Verification items for this drawing (mm, ordinates from the low corner). A direction names the side the tool comes from. Round coordinates to 2 decimals unless told otherwise and drop trailing zeros. Order: outer loops, then holes, each group sorted by start corner. A loop starts at its lowest first (then second) coordinate and runs counter-clockwise, first axis right, second up. Notation, with made-up numbers: (-24.75, 0) -> (25.25, 0) arc R23 cw to (25.25, 17) -> close; hole circle Ø9 at (46.5, 23). An arc over 180 degrees is marked (long way). Answer in a Markdown table with one row per item.
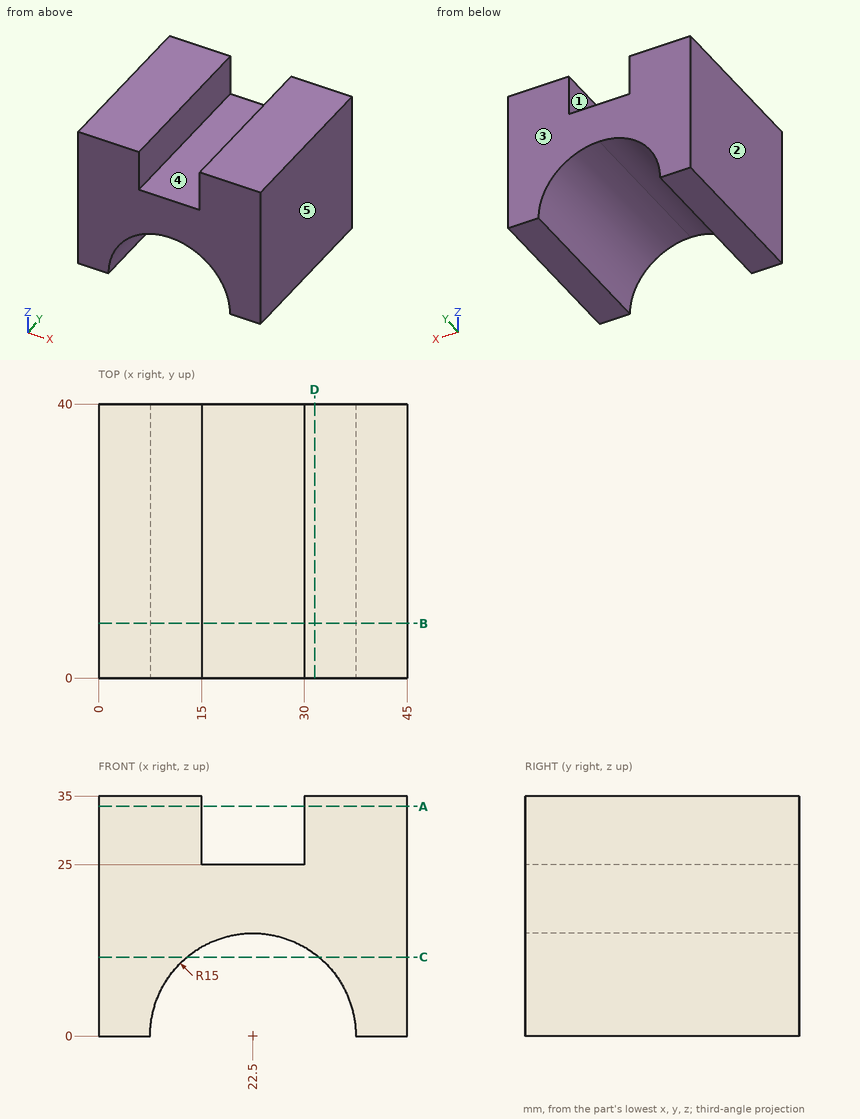
Item 1: Cross-section at D-D (x = 31.5). Record the boundary of the cut face in (y, z), and give its area (3 significant figures).
Result sheet:
| item | result |
|---|---|
| outline | (0, 12) -> (40, 12) -> (40, 35) -> (0, 35) -> close |
| area | 920 mm^2 |
Item 2: Depth check by flat-ended pin: P1, Ø8, axis at x = 35, y = 23, coming from the -Z side; P2, Ø6, axis at x = 14.5, y = 24, coming from the -Z side. Enter the tip coordinate at first touch or a pass-through.
Result sheet:
| item | result |
|---|---|
| P1 | stops at z = 0 |
| P2 | stops at z = 10.2 |
Item 3: Cross-section at A-A (z = 33.5). Record the boundary of the cut face in (x, y), and give its area (3 significant figures).
Result sheet:
| item | result |
|---|---|
| outline | (0, 0) -> (15, 0) -> (15, 40) -> (0, 40) -> close; (30, 0) -> (45, 0) -> (45, 40) -> (30, 40) -> close |
| area | 1,200 mm^2 |
Item 4: Cross-section at B-B (y = 8). Record the boundary of the cut face in (x, z).
Result sheet:
| item | result |
|---|---|
| outline | (0, 0) -> (7.5, 0) arc R15 cw to (22.5, 15) arc R15 cw to (37.5, 0) -> (45, 0) -> (45, 35) -> (30, 35) -> (30, 25) -> (15, 25) -> (15, 35) -> (0, 35) -> close |
Item 5: Scan lines: line 1 (X direction, y = 27.5, z = 31); line 2 (X direction, y = 22, z = 7.5); line 3 (Z direction, x = 23, y = 20). Record each from-to range of solid material in increasing order. Write a range as [from, to].
Result sheet:
| item | result |
|---|---|
| line 1 | x = [0, 15], [30, 45] |
| line 2 | x = [0, 9.51], [35.49, 45] |
| line 3 | z = [14.99, 25] |
Item 6: Mould release check, pull along X, two halves, no side actions. Record for the marked faces 3, 4 and 5: pulls with the +X half, pulls with the -X half, needs draft (parallel to the pull), parting line crosses it, or undercut.
Result sheet:
| item | result |
|---|---|
| face 3 | needs draft |
| face 4 | undercut |
| face 5 | pulls with the +X half |
Item 7: Set-up check for the marked faces 1 and 2: record each of +Z, -Z, +X, -X, +Y, -Y from which the full face is reachable in a straight line by a thin tool's end or side.
Result sheet:
| item | result |
|---|---|
| face 1 | +Z, +Y, -Y |
| face 2 | +Z, -Z, -X, +Y, -Y |
Item 8: Cross-section at C-C (z = 11.5). Record the boundary of the cut face in (x, y), and give its area (3 significant figures).
Result sheet:
| item | result |
|---|---|
| outline | (0, 0) -> (12.87, 0) -> (12.87, 40) -> (0, 40) -> close; (32.13, 0) -> (45, 0) -> (45, 40) -> (32.13, 40) -> close |
| area | 1,030 mm^2 |
